from build123d import *

# Parameters (mm, degrees)
F1_DEPTH = 5
F2_R     = 1.75
F3_DEPTH = 5
F5_DEPTH = 5


with BuildPart() as f1:
    # F0 (on Top) → F1 (new body)
    with BuildSketch(Plane.XY):
        with BuildLine():
            Line((-29, -28), (29, -28))
            ThreePointArc((29, -28), (31.474874, -26.974874), (32.5, -24.5))
            Line((32.5, -24.5), (32.5, 24.5))
            ThreePointArc((32.5, 24.5), (31.474874, 26.974874), (29, 28))
            Line((29, 28), (-29, 28))
            ThreePointArc((-29, 28), (-31.474874, 26.974874), (-32.5, 24.5))
            Line((-32.5, 24.5), (-32.5, -24.5))
            ThreePointArc((-32.5, -24.5), (-31.474874, -26.974874), (-29, -28))
        make_face()
    extrude(amount=F1_DEPTH)

    # F2 (on face) → F3 (cut)
    with BuildSketch(Plane.XY.offset(5)):
        with Locations((-29, 24.5)):
            Circle(F2_R)
        with Locations((29, 24.5)):
            Circle(F2_R)
        with Locations((29, -24.5)):
            Circle(F2_R)
        with Locations((-29, -24.5)):
            Circle(F2_R)
    extrude(amount=-F3_DEPTH, mode=Mode.SUBTRACT)

    # F4 (on face) → F5 (cut)
    with BuildSketch(Plane.XY.offset(5)):
        with BuildLine():
            Line((22.065871, 23), (-22.065871, 23))
            ThreePointArc((-22.065871, 23), (-23.98342, 19.48342), (-27.5, 17.565871))
            Line((-27.5, 17.565871), (-27.5, -17.565871))
            ThreePointArc((-27.5, -17.565871), (-23.98342, -19.48342), (-22.065871, -23))
            Line((-22.065871, -23), (22.065871, -23))
            ThreePointArc((22.065871, -23), (23.98342, -19.48342), (27.5, -17.565871))
            Line((27.5, -17.565871), (27.5, 17.565871))
            ThreePointArc((27.5, 17.565871), (23.98342, 19.48342), (22.065871, 23))
        make_face()
    extrude(amount=-F5_DEPTH, mode=Mode.SUBTRACT)


solid = f1.part
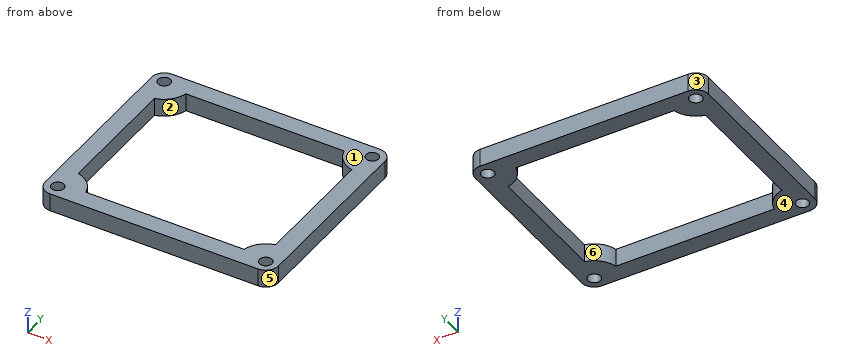
Read the model definition and answer for the solid it produces. Units are mm, in the model's axes. Face numbers are marked on the shaded views. A direction names the side the tool comes from. Round coordinates to 2 decimals unless told otherwise and drop trailing zeros. Write each loop counter-clockwise with the first axis right and the second up, starting at its lowest first coordinate (ties: lowest second). Pieces come first, ordered by that corner, then holes.
1. Which of the six approach directions +Z, -Z, +X, -X, +Y, -Y give full straight-line access (tool end or side, diameter ignored) to the marked faces 1 and 2?
2. The part is cut by section B-B, the plane z = 1.4. Determine the outline of the cut face in (x, y), then the cut area to 3 significant figures.
3. The part is cut by section C-C, the plane y = -21. Determine the outline of the cut face in (x, z).
4. The part is cut by section A-A, the plane x = -17. Determine the outline of the cut face in (y, z).
5. Determine the mould class of the marked faces 3, 4, 5 and 6 for opening direction X: pulls with the +X half, pulls with the -X half, needs draft (parallel to the pull), parting line crosses it, or undercut.
6. Straight lines are drawn through the part: L1, parallel to Y at x = 29, z = 3.6; L2, parallel to X at y = -13, z = 3.1; L3, parallel to Y at x = -19, z = 3.8. For each, find the intervals that lie inside material, in ascending order.
Values:
1. face 1: +Z, +X, -X, +Y, -Y
1. face 2: +Z, -Z
2. outline: (-32.5, -24.5) arc R3.5 ccw to (-29, -28) - (29, -28) arc R3.5 ccw to (32.5, -24.5) - (32.5, 24.5) arc R3.5 ccw to (29, 28) - (-29, 28) arc R3.5 ccw to (-32.5, 24.5) - close; hole circle Ø3.5 at (-29, -24.5); hole circle Ø3.5 at (-29, 24.5); hole (-27.5, -17.57) arc R7.09 cw to (-22.07, -23) - (22.07, -23) arc R7.09 cw to (27.5, -17.57) - (27.5, 17.57) arc R7.09 cw to (22.07, 23) - (-22.07, 23) arc R7.09 cw to (-27.5, 17.57) - close; hole circle Ø3.5 at (29, -24.5); hole circle Ø3.5 at (29, 24.5)
2. area: 1,140 mm2
3. outline: (-32.5, 0) - (-22.83, 0) - (-22.83, 5) - (-32.5, 5) - close; (22.83, 0) - (32.5, 0) - (32.5, 5) - (22.83, 5) - close
4. outline: (-28, 0) - (-23, 0) - (-23, 5) - (-28, 5) - close; (23, 0) - (28, 0) - (28, 5) - (23, 5) - close
5. face 3: pulls with the -X half
5. face 4: needs draft
5. face 5: pulls with the +X half
5. face 6: undercut
6. L1: y = -28 to -26.25, -22.75 to 22.75, 26.25 to 28
6. L2: x = -32.5 to -27.5, 27.5 to 32.5
6. L3: y = -28 to -23, 23 to 28
